```python
from build123d import *

# Parameters (mm, degrees)
CROQUIS1_W              = 61
CROQUIS1_H              = 100
SALIENTE_EXTRUIR1_DEPTH = 3
CROQUIS7_W              = 19.5
CROQUIS7_H              = 40.5
SALIENTE_EXTRUIR4_DEPTH = 3
CROQUIS17_W             = 61
CROQUIS17_H             = 3.5
CORTAR_EXTRUIR10_DEPTH  = 10
CROQUIS2_R              = 1.1
CROQUIS2_R_2            = 1.05
CORTAR_EXTRUIR1_DEPTH   = 3
CROQUIS8_W              = 13
CROQUIS8_H              = 23
CORTAR_EXTRUIR3_DEPTH   = 10
CROQUIS3_R              = 1.6
CORTAR_EXTRUIR2_DEPTH   = 82.665476182
CROQUIS12_R             = 1.6
CORTAR_EXTRUIR6_DEPTH   = 82.665476182
CORTAR_EXTRUIR7_DEPTH   = 82.665476182
REDONDEO2_R             = 4
REDONDEO3_R             = 2
CORTAR_EXTRUIR8_DEPTH   = 10
MATRIZ_CRV1_OUTLINE_W   = 5.1
MATRIZ_CRV1_OUTLINE_H   = 3.1
MATRIZ_CRV1_DEPTH       = 3
CROQUIS16_W             = 3.1
CROQUIS16_H             = 4.1
CROQUIS16_H_2           = 5.1
CORTAR_EXTRUIR9_DEPTH   = 3
CORTAR_EXTRUIR13_DEPTH  = 82.665476326
CROQUIS18_W             = 10.1
CROQUIS18_H             = 3.1
CORTAR_EXTRUIR11_DEPTH  = 10
CROQUIS9_R              = 1
CROQUIS9_W              = 11.6
CROQUIS9_H              = 5.7
CORTAR_EXTRUIR4_DEPTH   = 10


# Read off the part's stored shape, not the designer's step: Matriz Crv1
with BuildPart() as part:
    # Croquis1 → Saliente-Extruir1 (new body)
    with BuildSketch(Plane(origin=(0, 0, 0), x_dir=(1, 0, 0), z_dir=(0, 1, 0))):
        with Locations((0, -18)):
            Rectangle(CROQUIS1_W, CROQUIS1_H)
    extrude(amount=SALIENTE_EXTRUIR1_DEPTH)

    # Croquis7 → Saliente-Extruir4 (add, through all)
    with BuildSketch(Plane(origin=(0, 3, 0), x_dir=(1, 0, 0), z_dir=(0, 1, 0))):
        with BuildLine():
            Line((-30.5, 24), (-30.5, 32))
            Line((-30.5, 32), (30.5, 32))
            Line((30.5, 32), (30.5, 24))
            Line((30.5, 24), (50, 24))
            Line((50, 24), (50, 30))
            ThreePointArc((50, 30), (0, 42.950013881), (-50, 30))
            Line((-50, 30), (-50, 24))
            Line((-50, 24), (-30.5, 24))
        make_face()
        with Locations((-40.25, -44.25)):
            Rectangle(CROQUIS7_W, CROQUIS7_H)
        with Locations((40.25, -44.25)):
            Rectangle(CROQUIS7_W, CROQUIS7_H)
    extrude(amount=-SALIENTE_EXTRUIR4_DEPTH)

    # Croquis17 → Cortar-Extruir10 (cut)
    with BuildSketch(Plane(origin=(0, 3, 0), x_dir=(1, 0, 0), z_dir=(0, 1, 0))):
        with Locations((0, -66.25)):
            Rectangle(CROQUIS17_W, CROQUIS17_H)
    extrude(amount=-CORTAR_EXTRUIR10_DEPTH, mode=Mode.SUBTRACT)

    # Croquis2 → Cortar-Extruir1 (cut)
    with BuildSketch(Plane(origin=(0, 3, 0), x_dir=(1, 0, 0), z_dir=(0, 1, 0))):
        with Locations(Location((23.5, 9, 0), (0, 0, 270))):
            Circle(CROQUIS2_R)
        with Locations(Location((23.5, -9, 0), (0, 0, 270))):
            Circle(CROQUIS2_R)
        with Locations(Location((-23.5, 9, 0), (0, 0, 270))):
            Circle(CROQUIS2_R)
        with Locations(Location((-23.5, -9, 0), (0, 0, 270))):
            Circle(CROQUIS2_R)
        with Locations(Location((-8, -52, 0), (0, 0, 270))):
            Circle(CROQUIS2_R_2)
        with Locations(Location((8, -52, 0), (0, 0, 270))):
            Circle(CROQUIS2_R_2)
    extrude(amount=-CORTAR_EXTRUIR1_DEPTH, mode=Mode.SUBTRACT)

    # Croquis8 → Cortar-Extruir3 (cut)
    with BuildSketch(Plane(origin=(0, 3, 0), x_dir=(1, 0, 0), z_dir=(0, 1, 0))):
        with Locations((0, 21)):
            Rectangle(CROQUIS8_W, CROQUIS8_H)
    extrude(amount=-CORTAR_EXTRUIR3_DEPTH, mode=Mode.SUBTRACT)

    # Croquis3 → Cortar-Extruir2 (cut, through all)
    with BuildSketch(Plane(origin=(0, 3, 0), x_dir=(1, 0, 0), z_dir=(0, 1, 0))):
        with Locations(Location((-11, 12, 0), (0, 0, 270))):
            Circle(CROQUIS3_R)
        with Locations(Location((11, 12, 0), (0, 0, 270))):
            Circle(CROQUIS3_R)
        with Locations(Location((-33.5, -45, 0), (0, 0, 270))):
            Circle(CROQUIS3_R)
        with Locations(Location((33.5, -45, 0), (0, 0, 270))):
            Circle(CROQUIS3_R)
        with BuildLine():
            Line((-1.6, -9), (-1.6, -5))
            ThreePointArc((-1.6, -5), (0, -3.4), (1.6, -5))
            Line((1.6, -5), (1.6, -9))
            ThreePointArc((1.6, -9), (0, -10.6), (-1.6, -9))
        make_face()
    extrude(amount=-CORTAR_EXTRUIR2_DEPTH, mode=Mode.SUBTRACT)

    # Croquis12 → Cortar-Extruir6 (cut, through all)
    with BuildSketch(Plane(origin=(0, 3, 0), x_dir=(1, 0, 0), z_dir=(0, 1, 0))):
        with Locations(Location((-18, 29.5, 0), (0, 0, 270))):
            Circle(CROQUIS12_R)
        with Locations(Location((18, 29.5, 0), (0, 0, 270))):
            Circle(CROQUIS12_R)
    extrude(amount=-CORTAR_EXTRUIR6_DEPTH, mode=Mode.SUBTRACT)

    # Croquis14 → Cortar-Extruir7 (cut, through all)
    with BuildSketch(Plane(origin=(0, 3, 0), x_dir=(1, 0, 0), z_dir=(0, 1, 0))):
        with BuildLine():
            Line((-50, -26), (-50, -64.5))
            Line((-50, -64.5), (-28, -64.5))
            add(Edge.make_bspline(
                [(-50, -26), (-50, -38), (-40, -64.5), (-28, -64.5)],
                knots=[0, 0, 0, 0, 1, 1, 1, 1], degree=3))
        make_face()
    cortar_extruir7 = extrude(amount=-CORTAR_EXTRUIR7_DEPTH, mode=Mode.SUBTRACT)

    # Redondeo2
    redondeo2_edges = [part.edges().sort_by_distance(p)[0] for p in [
        (30.5, 1.5, -24),
        (-30.5, 1.5, -24),
        (-30.5, 1.5, 24),
        (30.5, 1.5, 24),
    ]]
    fillet(redondeo2_edges, radius=REDONDEO2_R)

    # Redondeo3
    redondeo3_edges = [part.edges().sort_by_distance(p)[0] for p in [
        (-50, 1.5, -30),
        (50, 1.5, -30),
        (50, 1.5, -24),
        (-50, 1.5, -24),
        (-50, 1.5, 24),
        (50, 1.5, 24),
    ]]
    fillet(redondeo3_edges, radius=REDONDEO3_R - 0.0001)  # a hair under: the kernel refuses the full size

    # Croquis15 → Cortar-Extruir8 (cut)
    with BuildSketch(Plane(origin=(0, 3, 0), x_dir=(1, 0, 0), z_dir=(0, 1, 0))):
        Polygon((-38.239465907, 29.620233281), (-33.497496925, 31.497393416), (-34.638515831, 34.379766719), (-39.380484813, 32.502606584), align=None)
    extrude(amount=-CORTAR_EXTRUIR8_DEPTH, mode=Mode.SUBTRACT)

    # Matriz Crv1 outline → Matriz Crv1 (cut)
    with BuildSketch(Plane(origin=(0, 0, 0), x_dir=(1, 0, 0), z_dir=(0, 1, 0))):
        Polygon((39.380484813, 32.502606584), (34.638515831, 34.379766719), (33.497496925, 31.497393416), (38.239465907, 29.620233281), align=None)
        Polygon((27.471913222, 36.707954041), (22.532090053, 37.976081424), (21.761267526, 34.973443811), (26.701090695, 33.705316428), align=None)
        Polygon((15.130226298, 39.387839944), (10.070428962, 40.026941594), (9.68195541, 36.951378508), (14.741752746, 36.312276858), align=None)
        with Locations((0, 38.950013881)):
            Rectangle(MATRIZ_CRV1_OUTLINE_W, MATRIZ_CRV1_OUTLINE_H)
        Polygon((-10.070428962, 40.026941594), (-15.130226298, 39.387839944), (-14.741752746, 36.312276858), (-9.68195541, 36.951378508), align=None)
        Polygon((-22.532090053, 37.976081424), (-27.471913222, 36.707954041), (-26.701090695, 33.705316428), (-21.761267526, 34.973443811), align=None)
    extrude(amount=MATRIZ_CRV1_DEPTH, mode=Mode.SUBTRACT)

    # Croquis16 → Cortar-Extruir9 (cut)
    with BuildSketch(Plane(origin=(0, 3, 0), x_dir=(1, 0, 0), z_dir=(0, 1, 0))):
        with Locations((-44.5, 27.885018263)):
            Rectangle(CROQUIS16_W, CROQUIS16_H)
        with Locations((-44.5, -29.5)):
            Rectangle(CROQUIS16_W, CROQUIS16_H_2)
    cortar_extruir9 = extrude(amount=-CORTAR_EXTRUIR9_DEPTH, mode=Mode.SUBTRACT)

    # Croquis19 → Cortar-Extruir13 (cut, through all)
    with BuildSketch(Plane(origin=(0, 3, 0), x_dir=(1, 0, 0), z_dir=(0, 1, 0))):
        Polygon((-40.014205747, -42.823860895), (-41.724634952, -38.019234798), (-44.645093952, -39.058907452), (-42.934664747, -43.863533549), align=None)
        Polygon((-38.866197007, -52.280851683), (-35.970669214, -56.479175015), (-33.418747189, -54.719148317), (-36.314274981, -50.520824985), align=None)
    cortar_extruir13 = extrude(amount=-CORTAR_EXTRUIR13_DEPTH, mode=Mode.SUBTRACT)

    # Simetría1: Cortar-Extruir7, Cortar-Extruir9, Cortar-Extruir13 across plane
    add(cortar_extruir7.mirror(Plane(origin=(0, 0, 0), x_dir=(0, 0, 1), z_dir=(1, 0, 0))), mode=Mode.SUBTRACT)
    add(cortar_extruir9.mirror(Plane(origin=(0, 0, 0), x_dir=(0, 0, 1), z_dir=(1, 0, 0))), mode=Mode.SUBTRACT)
    add(cortar_extruir13.mirror(Plane(origin=(0, 0, 0), x_dir=(0, 0, 1), z_dir=(1, 0, 0))), mode=Mode.SUBTRACT)

    # Croquis18 → Cortar-Extruir11 (cut)
    with BuildSketch(Plane(origin=(0, 3, 0), x_dir=(1, 0, 0), z_dir=(0, 1, 0))):
        with Locations((0, -60.5)):
            Rectangle(CROQUIS18_W, CROQUIS18_H)
        with Locations((20, -60.5)):
            Rectangle(CROQUIS18_W, CROQUIS18_H)
        with Locations((-20, -60.5)):
            Rectangle(CROQUIS18_W, CROQUIS18_H)
    extrude(amount=-CORTAR_EXTRUIR11_DEPTH, mode=Mode.SUBTRACT)

    # Croquis9 → Cortar-Extruir4 (cut)
    with BuildSketch(Plane(origin=(0, 3, 0), x_dir=(1, 0, 0), z_dir=(0, 1, 0))):
        with Locations(Location((11, 20.5, 0), (0, 0, 270))):
            Circle(CROQUIS9_R)
        with Locations(Location((26, 20.5, 0), (0, 0, 270))):
            Circle(CROQUIS9_R)
        with Locations((18.5, 20.5)):
            Rectangle(CROQUIS9_W, CROQUIS9_H)
    extrude(amount=-CORTAR_EXTRUIR4_DEPTH, mode=Mode.SUBTRACT)


solid = part.part
```
Input: part model. Units: mm. Frame: model coordinates. A direction names the side the tool comes from. Round coordinates to 2 decimals unless told otherwise and drop trailing zeros. Loops run counter-clockwise (first coordinate to the right, second up) from the corner with the lowest first, then second, coordinate; pieces in that order, holes last. Notation, with made-up numbers: (-24.75, 1.5) -> (26.25, 1.5) arc R23 ccw to (26.25, 30.5) -> close; hole circle Ø4 at (10.25, 3). An arc over 180 degrees is marked (long way). Use one line per item in the form item = value. Start each with the question number.
Item 1: Section query C-C on y = 2.05. Count the separate pieces of the cut face and the enclosed holes in it, then the cut area to 3 significant figures.
Item 2: Section query B-B on x = 18. Return the cut outline in (y, z) (3 decimals).
Item 3: Mould query, pull axis X, two halves, no side actions, for faces 3 (the face through (0.714, 1.521, -42.948)), 4 (the face through (50, 2, -27)), 5 (the face through (-42.95, 2, -28)). Classes: pulls with the +X half, pulls with the -X half, needs draft (parallel to the pull), parting line crosses it, or undercut.
Item 4: Material intervals for L1, parallel to X at y = 0.65, z = -12; L2, parallel to X at y = 2.3, z = 9; L3, parallel to X at y = 2.55, z = -18.5, sorted ascending. Write a range as from..to.
Item 5: Section query A-A on z = -16. Return the cut outline in (x, y).
Item 6: Contact query for flat-ended pins moving along their axis: pin 1 Ø1 at (y, z) = (2, -14.5) entering from -X; pin 2 Ø3.5 at (x, z) = (18, -29.5) entering from -Y; pin 3 Ø1.9 at (x, z) = (11, -12) entering from -Y. Output: stop coordinate, or through.
Item 7: Set-up query: faces 1 (the face through (41, 2, 24)), 2 (the face through (41.49, 1.52, 43.35)). Return all of +Z, -Z, +X, -X, +Y, -Y with unobstructed straight access to the full face (end or side cutting, diameter ignored); none if empty.
Ans:
q1.separate_pieces = 1
q1.enclosed_holes = 35
q1.area = 7,220 mm^2
q2.outline = (0, -41.365) -> (3, -41.365) -> (3, -31.1) -> (0, -31.1) -> close; (0, -27.9) -> (3, -27.9) -> (3, -23.35) -> (0, -23.35) -> close; (0, -17.65) -> (3, -17.65) -> (3, 58.95) -> (0, 58.95) -> close; (0, 62.05) -> (3, 62.05) -> (3, 64.5) -> (0, 64.5) -> close
q3.face_3 = parting line crosses it
q3.face_4 = pulls with the +X half
q3.face_5 = undercut
q4.L1 = -30.5..-12.6, -9.4..-6.5, 6.5..9.4, 12.6..30.5
q4.L2 = -30.5..-24.6, -22.4..-1.6, 1.6..22.4, 24.6..30.5
q4.L3 = -30.5..-6.5, 6.5..12.7, 24.3..30.5
q5.outline = (-30.5, 0) -> (-6.5, 0) -> (-6.5, 3) -> (-30.5, 3) -> close; (6.5, 0) -> (30.5, 0) -> (30.5, 3) -> (6.5, 3) -> close
q6.pin_1 = -30.5
q6.pin_2 = 0
q6.pin_3 = through
q7.face_1 = +X, +Y, -Y
q7.face_2 = +Y, -Y
